CAD build for the part. Positions are in the model's coordinates, mm. Round coordinates to 2 decimals unless told otherwise and drop trailing zeros. Loops run counter-clockwise (first coordinate to the right, second up) from the corner with the lowest first, then second, coordinate; pieces in that order, holes last. Notation, with made-up numbers: M 17.25,11.25 L 73.25,11.25 A14 cw 73.25,16.25 Z; hole C 21,-4 d8. An arc over 180 degrees is marked long. Use a Markdown table: item, result. Add a question column.
(1) Band-saw the part on D-D, the plane y = -18. Write the cut outline in (x, z), and give its area (3 significant figures).
(2) Band-saw the part on C-C, the plane z = 16. Write the cut outline in (x, y), and give its area (3 significant figures).
(3) Flat gauge pins, fed straight in: P1, Ø2, axis at x = -22, z = 12.5, coming from the +Y side; P2, Ø1.8, axis at y = -15.5, z = 3, coming from the +X side; P3, Ø1.1, axis at y = 15.5, z = 5, coming from the +X side. Where does each tip first touch, or does it go through?
(4) Wall check: L1, parallel to Y at x = 0, z = 8.25; L2, parallel to Y at x = -14.5, z = 7; L3, parallel to Y at x = 18, z = 4.75. Give the ranges that are in metal, low to high.
(5) Band-saw the part on A-A, the plane x = 0. Write the cut outline in (y, z).
(6) Two-plate mould, pull along X, no slides. Class faces 1 (the face through (-14.9, -14.8, 5.6)), 2 (the face through (21.77, -34.15, 9.86)): released by +X, released by -X, zero draft, split by the parting line, or undercut.
Autodesk Inventor part; units mm, degrees
sketch "Sketch1" plane through (0, 0, 0) normal (0, 0, 1) x (1, 0, 0)
  circle A0 centre (0, 0) radius 40.5
  dimension "d0" = 81
extrude "Extrusion1" add sketch "Sketch1" along normal blind 20
sketch "Sketch2" plane through (0, 0, 20) normal (0, 0, 1) x (1, 0, 0)
  circle A0 centre (0, 0) radius 22
  dimension "d3" = 44
extrude "Extrusion2" cut sketch "Sketch2" against normal blind 9
sketch "Sketch3" plane through (0, 0, 11) normal (0, 0, 1) x (1, 0, 0)
  circle A0 centre (0, 18) radius 2
  circle A1 centre (-18, 0) radius 2
  circle A2 centre (0, -18) radius 2
  circle A3 centre (18, 0) radius 2
  point P0 (0, 0)
  dimension "d6" = 4
  dimension "d7" = 18
  dimension "d10" = 360
extrude "Extrusion3" cut sketch "Sketch3" against normal blind 12.75
sketch "Sketch4" plane through (0, 0, 11) normal (0, 0, 1) x (1, 0, 0)
  arc A0 (-4.5165, 17.448) -> (-8.8542, 19.2414) centre (-7.5165, 16.3345) ccw
  arc A1 (-8.8542, 19.2414) -> (-19.0977, 9.16) centre (0, 0) ccw
  arc A2 (-14.1333, 4.5) -> (-11.4833, 6.0938) centre (-14.1333, 7.5) ccw
  line L0 (-4.5, 14.1333) -> (-4.5, 16.3631)
  arc A3 (-4.5, 16.3631) -> (-8.75, 19.0902) centre (-7.5, 16.3631) ccw
  arc A4 (-6.0938, 11.4833) -> (-4.5, 14.1333) centre (-7.5, 14.1333) ccw
  arc A5 (-6.0938, 11.4833) -> (-11.4833, 6.0938) centre (0, 0) ccw
  arc A6 (-8.8542, 19.2414) -> (-19.2547, 8.8254) centre (0, 0) ccw
  arc A7 (-8.75, 19.0902) -> (-19.0902, 8.75) centre (0, 0) ccw
  arc A8 (-19.0902, 8.75) -> (-16.3631, 4.5) centre (-16.3631, 7.5) ccw
  line L1 (-16.3631, 4.5) -> (-14.1333, 4.5)
  arc A9 (-11.4833, -6.0938) -> (-14.1333, -4.5) centre (-14.1333, -7.5) ccw
  arc A10 (-4.5, -14.1333) -> (-6.0938, -11.4833) centre (-7.5, -14.1333) ccw
  arc A11 (-11.4833, -6.0938) -> (-6.0938, -11.4833) centre (0, 0) ccw
  line L2 (-14.1333, -4.5) -> (-16.3631, -4.5)
  line L3 (-4.5, -16.3631) -> (-4.5, -14.1333)
  arc A12 (-16.3631, -4.5) -> (-19.0902, -8.75) centre (-16.3631, -7.5) ccw
  arc A13 (-17.448, -4.5165) -> (-19.2414, -8.8542) centre (-16.3345, -7.5165) ccw
  arc A14 (-8.75, -19.0902) -> (-4.5, -16.3631) centre (-7.5, -16.3631) ccw
  arc A15 (-19.0902, -8.75) -> (-8.75, -19.0902) centre (0, 0) ccw
  arc A16 (-19.2414, -8.8542) -> (-9.16, -19.0977) centre (0, 0) ccw
  arc A17 (-19.2414, -8.8542) -> (-8.8254, -19.2547) centre (0, 0) ccw
  arc A18 (6.0938, -11.4833) -> (4.5, -14.1333) centre (7.5, -14.1333) ccw
  arc A19 (14.1333, -4.5) -> (11.4833, -6.0938) centre (14.1333, -7.5) ccw
  arc A20 (6.0938, -11.4833) -> (11.4833, -6.0938) centre (0, 0) ccw
  line L4 (4.5, -14.1333) -> (4.5, -16.3631)
  line L5 (16.3631, -4.5) -> (14.1333, -4.5)
  arc A21 (4.5, -16.3631) -> (8.75, -19.0902) centre (7.5, -16.3631) ccw
  arc A22 (4.5165, -17.448) -> (8.8542, -19.2414) centre (7.5165, -16.3345) ccw
  arc A23 (19.0902, -8.75) -> (16.3631, -4.5) centre (16.3631, -7.5) ccw
  arc A24 (8.75, -19.0902) -> (19.0902, -8.75) centre (0, 0) ccw
  arc A25 (8.8542, -19.2414) -> (19.0977, -9.16) centre (0, 0) ccw
  arc A26 (8.8542, -19.2414) -> (19.2547, -8.8254) centre (0, 0) ccw
  arc A27 (11.4833, 6.0938) -> (14.1333, 4.5) centre (14.1333, 7.5) ccw
  arc A28 (4.5, 14.1333) -> (6.0938, 11.4833) centre (7.5, 14.1333) ccw
  arc A29 (11.4833, 6.0938) -> (6.0938, 11.4833) centre (0, 0) ccw
  line L6 (14.1333, 4.5) -> (16.3631, 4.5)
  line L7 (4.5, 16.3631) -> (4.5, 14.1333)
  arc A30 (16.3631, 4.5) -> (19.0902, 8.75) centre (16.3631, 7.5) ccw
  arc A31 (17.448, 4.5165) -> (19.2414, 8.8542) centre (16.3345, 7.5165) ccw
  arc A32 (8.75, 19.0902) -> (4.5, 16.3631) centre (7.5, 16.3631) ccw
  arc A33 (19.0902, 8.75) -> (8.75, 19.0902) centre (0, 0) ccw
  arc A34 (19.2414, 8.8542) -> (9.16, 19.0977) centre (0, 0) ccw
  arc A35 (19.2414, 8.8542) -> (8.8254, 19.2547) centre (0, 0) ccw
  point P0 (41.0732, 32.7294)
  point P1 (-17.4931, 4.4714)
  point P2 (-16.3796, 7.4714)
  point P3 (-7.4714, -16.3796)
  point P4 (-4.4714, -17.4931)
  point P5 (16.3796, -7.4714)
  point P6 (17.4931, -4.4714)
  point P7 (7.4714, 16.3796)
  point P8 (4.4714, 17.4931)
  dimension "d16" = 360
extrude "Extrusion4" cut sketch "Sketch4" against normal blind 12.75
ref_plane "Work Plane1" through (40.7, 0, 0) normal (1, 0, 0) x (0, 1, 0)
properties part number "MotorHousing" material "Plastic, Opaque White"
Return value:
| question | item | result |
|---|---|---|
| 1 | outline | M -36.28,0 L -10.82,0 L -10.82,11 L -12.65,11 L -12.65,20 L -36.28,20 Z; M -4.99,0 L -2,0 L -2,11 L -4.99,11 Z; M 2,0 L 4.99,0 L 4.99,11 L 2,11 Z; M 10.82,0 L 36.28,0 L 36.28,20 L 12.65,20 L 12.65,11 L 10.82,11 Z |
| 1 | area | 1,050 mm^2 |
| 2 | outline | C 0,0 d81; hole C 0,0 d44 |
| 2 | area | 3,630 mm^2 |
| 3 | P1 | y = 34.63 |
| 3 | P2 | x = 37.78 |
| 3 | P3 | x = 37.64 |
| 4 | L1 | -40.5 to -20, -16 to 16, 20 to 40.5 |
| 4 | L2 | -37.82 to -15.19, -4.5 to 4.5, 15.19 to 37.82 |
| 4 | L3 | -36.28 to -10.82, -4.99 to -2, 2 to 4.99, 10.82 to 36.28 |
| 5 | outline | M -40.5,0 L -20,0 L -20,11 L -22,11 L -22,20 L -40.5,20 Z; M -16,0 L 16,0 L 16,11 L -16,11 Z; M 20,0 L 40.5,0 L 40.5,20 L 22,20 L 22,11 L 20,11 Z |
| 6 | face 1 | undercut |
| 6 | face 2 | split by the parting line |
